from build123d import *

# Parameters (mm, degrees)
SKETCH_W        = 150
SKETCH_H        = 100
PAD_DEPTH       = 5
FILLET_R        = 5
SKETCH001_W     = 10
SKETCH001_H     = 10
PAD001_DEPTH    = 5
FILLET001_R     = 3
FILLET002_R     = 2
SKETCH002_R     = 2.5
POCKET_DEPTH    = 5
SKETCH003_W     = 60
SKETCH003_H     = 50
POCKET001_DEPTH = 5.001
SKETCH004_W     = 14
SKETCH004_H     = 7
POCKET002_DEPTH = 5.001
SKETCH005_W     = 16
SKETCH005_H     = 7
POCKET003_DEPTH = 2
SKETCH006_W     = 16
SKETCH006_H     = 9
POCKET004_DEPTH = 2
FILLET003_R     = 0.4


with BuildPart() as part:
    # Sketch → Pad (new body)
    with BuildSketch(Plane.XY):
        with Locations((75, 50)):
            Rectangle(SKETCH_W, SKETCH_H)
    extrude(amount=PAD_DEPTH)

    # Fillet
    fillet_edges = [part.edges().sort_by_distance(p)[0] for p in [
        (0, 0, 2.5),
        (150, 0, 2.5),
        (150, 100, 2.5),
        (0, 100, 2.5),
    ]]
    fillet(fillet_edges, radius=FILLET_R)

    # Sketch001 → Pad001 (new body)
    with BuildSketch(Plane.XY.offset(5)):
        with Locations((10, 10)):
            Rectangle(SKETCH001_W, SKETCH001_H)
        with Locations((140, 90)):
            Rectangle(SKETCH001_W, SKETCH001_H)
        with Locations((10, 90)):
            Rectangle(SKETCH001_W, SKETCH001_H)
        with Locations((140, 10)):
            Rectangle(SKETCH001_W, SKETCH001_H)
    extrude(amount=PAD001_DEPTH)

    # Fillet001
    fillet001_edges = [part.edges().sort_by_distance(p)[0] for p in [
        (5, 5, 7.5),
        (15, 5, 7.5),
        (5, 15, 7.5),
        (15, 15, 7.5),
        (5, 95, 7.5),
        (15, 95, 7.5),
        (5, 85, 7.5),
        (15, 85, 7.5),
        (135, 5, 7.5),
        (145, 5, 7.5),
        (145, 15, 7.5),
        (135, 85, 7.5),
        (145, 85, 7.5),
        (145, 95, 7.5),
        (135, 95, 7.5),
        (135, 15, 7.5),
    ]]
    fillet(fillet001_edges, radius=FILLET001_R)

    # Fillet002
    fillet002_edges = [part.edges().sort_by_distance(p)[0] for p in [
        (10, 15, 10),
        (140, 15, 10),
        (140, 95, 10),
        (10, 95, 10),
    ]]
    fillet(fillet002_edges, radius=FILLET002_R)

    # Sketch002 → Pocket (cut)
    with BuildSketch(Plane.XY.offset(5)):
        with Locations((56.8, 72.4)):
            Circle(SKETCH002_R)
        with Locations((127, 72.4)):
            Circle(SKETCH002_R)
        with Locations((56.8, 27.6)):
            Circle(SKETCH002_R)
        with Locations((127, 27.6)):
            Circle(SKETCH002_R)
    extrude(amount=-POCKET_DEPTH, mode=Mode.SUBTRACT)

    # Sketch003 → Pocket001 (cut, through all)
    with BuildSketch(Plane.XY.offset(5)):
        with Locations((91.9, 50)):
            Rectangle(SKETCH003_W, SKETCH003_H)
    extrude(amount=-POCKET001_DEPTH, mode=Mode.SUBTRACT)

    # Sketch004 → Pocket002 (cut, through all)
    with BuildSketch(Plane.XY.offset(5)):
        with Locations((27, 71.5)):
            Rectangle(SKETCH004_W, SKETCH004_H)
        with Locations((27, 28.5)):
            Rectangle(SKETCH004_W, SKETCH004_H)
    extrude(amount=-POCKET002_DEPTH, mode=Mode.SUBTRACT)

    # Sketch005 → Pocket003 (cut)
    with BuildSketch(Plane.XY.offset(5)):
        with Locations((27, 71.5)):
            Rectangle(SKETCH005_W, SKETCH005_H)
        with Locations((27, 28.5)):
            Rectangle(SKETCH005_W, SKETCH005_H)
    extrude(amount=-POCKET003_DEPTH, mode=Mode.SUBTRACT)

    # Sketch006 → Pocket004 (cut)
    with BuildSketch(Plane(origin=(0, 0, 0), x_dir=(1, 0, 0), z_dir=(0, 0, -1))):
        with Locations((27, -28.5)):
            Rectangle(SKETCH006_W, SKETCH006_H)
        with Locations((27, -71.5)):
            Rectangle(SKETCH006_W, SKETCH006_H)
    extrude(amount=-POCKET004_DEPTH, mode=Mode.SUBTRACT)

    # Fillet003
    fillet003_edges = [part.edges().sort_by_distance(p)[0] for p in [
        (34, 28.5, 3),
        (34, 28.5, 2),
        (20, 28.5, 3),
        (20, 28.5, 2),
        (20, 71.5, 3),
        (20, 71.5, 2),
        (34, 71.5, 3),
        (34, 71.5, 2),
    ]]
    fillet(fillet003_edges, radius=FILLET003_R)


solid = part.part
CAD build for the part. Positions are in the model's coordinates, mm. A direction names the side the tool comes from. Give positions to 0.01 mm unless a question says otherwise; leave off trailing zeros. Loops run counter-clockwise (first coordinate to the right, second up) from the corner with the lowest first, then second, coordinate; pieces in that order, holes last. Notation, with made-up numbers: M 51.5,-35.5 L 93.5,-35.5 A20 ccw 93.5,0.5 Z; hole C 48,-18 d5. An arc over 180 degrees is marked long. Answer in a Markdown table with one row per item. Add a question column.
Item 1: Probe probe 1 along Y at (x, z) = (31, 4.75); probe 2 along Y at (x, z) = (20, 1); probe 3 along X at (y, z) = (55.5, 0.75). List the from-to ranges inside material, lowest first.
Item 2: Band-saw the part on C-C on y = 27.6. Give the number of separate pieces and of enclosed holes in the cut face, then the cut area to 3 significant figures.
Item 3: Drop flat-ended pins along their axis: P1, Ø0.9, axis at x = 139.5, z = 7, coming from the +Y side; P2, Ø3.5, axis at x = 10, z = 6.5, coming from the +Y side; P3, Ø5, axis at x = 35.5, y = 44.5, coming from the +Z side; P4, Ø1.5, axis at x = 139.5, z = 6, coming from the -Y side. Give the stop position or say it passes through.
Item 4: Band-saw the part on D-D on x = 25. Give the cut face in (y, z).
Item 5: Tool access for faces 1 (the face through (140, 5, 6)), 2 (the face through (144.14, 14.1, 6.52)), 3 (the face through (140, 85, 6)), 4 (the face through (27, 24.8, 2)), 5 (the face through (135.9, 14.14, 6.52)): list every direction of +Z, -Z, +X, -X, +Y, -Y with a clear straight run to the whole face (end or side of a thin tool).
Item 6: Band-saw the part on A-A on x = 100.5. Give the cut face in (y, z), then the cut area to 3 significant figures.
Item 7: Band-saw the part on B-B on x = 127. Give the cut face in (y, z), then the cut area to 3 significant figures.
Item 8: Mould opens along Y. For faces 6 (the face through (129.31, 71.44, 2.54)), 7 (the face through (135.9, 94.14, 6.52)), 8 (the face through (145, 90, 6)) say: +Y half, -Y half, draft (parallel to the pull), parting line (faces both ways), or undercut.
Reply:
| question | item | result |
|---|---|---|
| 1 | probe 1 | y = 0 to 25, 32 to 68, 75 to 100 |
| 1 | probe 2 | y = 0 to 24, 33 to 67, 76 to 100 |
| 1 | probe 3 | x = 0 to 61.9, 121.9 to 150 |
| 2 | separate pieces | 5 |
| 2 | enclosed holes | 0 |
| 2 | area | 322 mm^2 |
| 3 | P1 | stops at y = 95 |
| 3 | P2 | stops at y = 100 |
| 3 | P3 | stops at z = 5 |
| 3 | P4 | stops at y = 5 |
| 4 | outline | M 0,0 L 24,0 L 24,2 L 25,2 L 25,5 L 0,5 Z; M 32,2 L 33,2 L 33,0 L 67,0 L 67,2 L 68,2 L 68,5 L 32,5 Z; M 75,2 L 76,2 L 76,0 L 100,0 L 100,5 L 75,5 Z |
| 5 | face 1 | +Z, +X, -X, -Y |
| 5 | face 2 | +Z, +X |
| 5 | face 3 | +Z, +X, -X |
| 5 | face 4 | -Z |
| 5 | face 5 | +Z |
| 6 | outline | M 0,0 L 25,0 L 25,5 L 0,5 Z; M 75,0 L 100,0 L 100,5 L 75,5 Z |
| 6 | area | 250 mm^2 |
| 7 | outline | M 0,0 L 25.1,0 L 25.1,5 L 0,5 Z; M 30.1,0 L 69.9,0 L 69.9,5 L 30.1,5 Z; M 74.9,0 L 100,0 L 100,5 L 74.9,5 Z |
| 7 | area | 450 mm^2 |
| 8 | face 6 | undercut |
| 8 | face 7 | +Y half |
| 8 | face 8 | draft |
